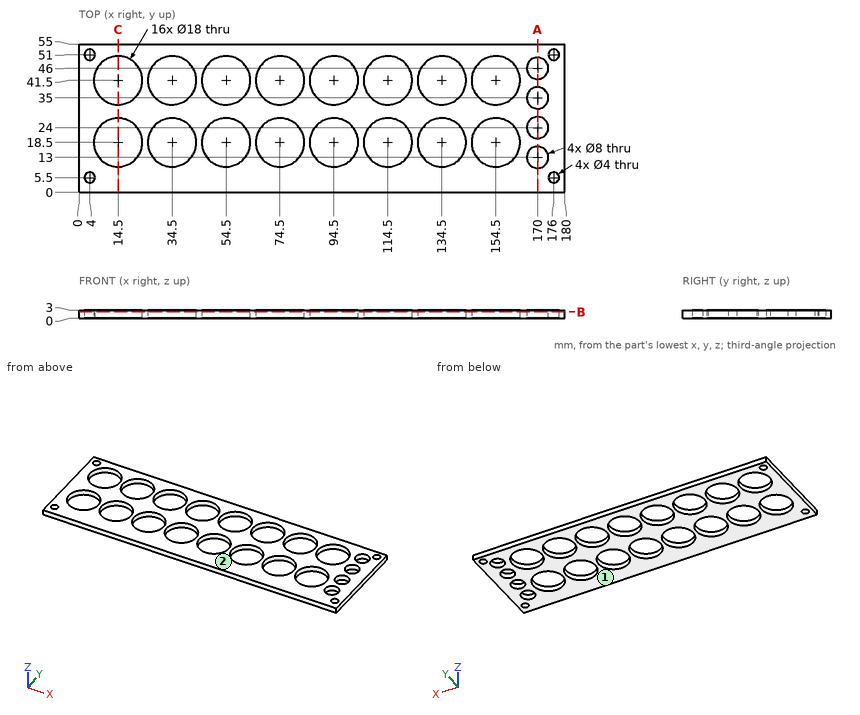
Can you work these out from the drawing? Everything is in mm from the part's minimum corner. Coordinates: 2 decimals unless noted, no trailing zeros. Loops run counter-clockwise (first coordinate to the right, second up) from the corner with the lowest first, then second, coordinate; pieces in that order, holes last.
1. If we mould it in two halves opening along Z, with no side actions, what happens to the marked faces 1 and 2? For each: pulls with the +Z half, pulls with the -Z half, needs draft (parallel to the pull), parting line crosses it, or undercut.
2. Imagine slicing it at A-A, the plane x = 170. Please give me the cut outline in (y, z), and give its area (3 significant figures).
3. Imagine slicing it at B-B, the plane z = 2.45. Count the separate pieces of the cut face and the enclosed holes in it, and give its area (3 significant figures).
4. Imagine slicing it at C-C, the plane x = 14.5. Please give me the cut outline in (y, z), and give its area (3 significant figures).
5. I need wall thicknesses on L1, parallel to Y at x = 154.5, z = 1.4; L2, parallel to Y at x = 121, z = 2.05. Which ranges of each line are inside material? Lowest first, please.
6. For P1, Ø11, axis at x = 74.5, y = 18.5, coming from the +Z side; P2, Ø23.5, axis at x = 14.5, y = 41.5, coming from the +Z side, each with a flat end and sliding along its axis, tell me the tip position at first contact or that it passes through.
Taken from the geometry:
1. face 1: pulls with the -Z half
1. face 2: pulls with the +Z half
2. outline: (0, 0) - (9, 0) - (9, 3) - (0, 3) - close; (17, 0) - (20, 0) - (20, 3) - (17, 3) - close; (28, 0) - (31, 0) - (31, 3) - (28, 3) - close; (39, 0) - (42, 0) - (42, 3) - (39, 3) - close; (50, 0) - (55, 0) - (55, 3) - (50, 3) - close
2. area: 69.0 mm2
3. separate pieces: 1
3. enclosed holes: 24
3. area: 5,580 mm2
4. outline: (0, 0) - (9.5, 0) - (9.5, 3) - (0, 3) - close; (27.5, 0) - (32.5, 0) - (32.5, 3) - (27.5, 3) - close; (50.5, 0) - (55, 0) - (55, 3) - (50.5, 3) - close
4. area: 57.0 mm2
5. L1: y = 0 to 9.5, 27.5 to 32.5, 50.5 to 55
5. L2: y = 0 to 12.28, 24.72 to 35.28, 47.72 to 55
6. P1: passes through
6. P2: stops at z = 3
